from build123d import *

# Parameters (mm, degrees)
BOSS_EXTRUDE1_DEPTH              = 20
SKETCH2_R                        = 5
CUT_EXTRUDE1_DEPTH               = 10
SKETCH3_R                        = 10
CUT_EXTRUDE2_DEPTH               = 10
F_10_8_10_8_DIAMETER_HOLE1_D     = 10.8
F_10_8_10_8_DIAMETER_HOLE1_DEPTH = 5
F_10_8_10_8_DIAMETER_HOLE1_TIP   = 3.244647343
F_6_6_6_6_DIAMETER_HOLE1_D       = 6.6


with BuildPart() as part:
    # Sketch1 → Boss-Extrude1 (new body)
    with BuildSketch(Plane.XY):
        Polygon((-17, 16.25), (-17, 26.75), (17, 26.75), (17, 16.25), (30, 16.25), (30, -16.25), (-30, -16.25), (-30, 16.25), align=None)
    extrude(amount=BOSS_EXTRUDE1_DEPTH)

    # Sketch2 → Cut-Extrude1 (cut)
    with BuildSketch(Plane.XY.offset(20)):
        with Locations((0, 8.75)):
            Circle(SKETCH2_R)
    extrude(amount=-CUT_EXTRUDE1_DEPTH, mode=Mode.SUBTRACT)

    # Sketch3 → Cut-Extrude2 (cut)
    with BuildSketch(Plane(origin=(0, 0, 0), x_dir=(-1, 0, 0), z_dir=(0, 0, -1))):
        with Locations((0, 8.75)):
            Circle(SKETCH3_R)
    extrude(amount=-CUT_EXTRUDE2_DEPTH, mode=Mode.SUBTRACT)

    # Ø10.8 (10.8) Diameter Hole1
    with Locations(Plane(origin=(0, 16.25, 0), x_dir=(1, 0, 0), z_dir=(0, 1, 0))):
        with Locations((-23, -10), (23, -10)):
            Hole(F_10_8_10_8_DIAMETER_HOLE1_D / 2, depth=F_10_8_10_8_DIAMETER_HOLE1_DEPTH)
            with Locations((0, 0, -(F_10_8_10_8_DIAMETER_HOLE1_DEPTH + F_10_8_10_8_DIAMETER_HOLE1_TIP / 2))):  # 118° drill point
                Cone(0, F_10_8_10_8_DIAMETER_HOLE1_D / 2, F_10_8_10_8_DIAMETER_HOLE1_TIP, mode=Mode.SUBTRACT)

    # Ø6.6 (6.6) Diameter Hole1 (through all)
    with Locations(Plane(origin=(0, 16.25, 0), x_dir=(1, 0, 0), z_dir=(0, 1, 0))):
        with Locations((-23, -10), (23, -10)):
            Hole(F_6_6_6_6_DIAMETER_HOLE1_D / 2)


solid = part.part
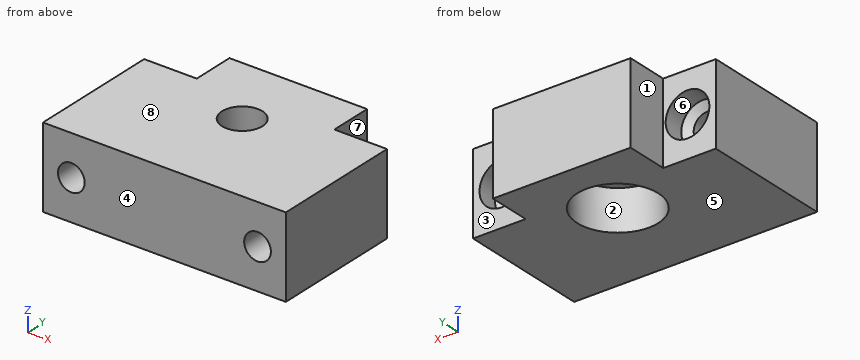
Read the model definition and answer for the solid it produces. Units are mm, in the model's axes. Face numbers are marked on the shaded views. A direction names the side the tool comes from. Give positions to 0.01 mm unless a question says otherwise; leave off trailing zeros. Write each loop counter-clockwise with the first axis right and the second up, starting at its lowest first coordinate (ties: lowest second). Pieces come first, ordered by that corner, then holes. Notation, with made-up numbers: (75.25, 9) - (107.25, 9) arc R19 ccw to (107.25, 25) - close; hole circle Ø4 at (80, -27.75). An arc over 180 degrees is marked (long way). Use CSV: the item, a comma, the result in double quotes. Start each with the question number.
Item 1: Flat-ended cylindrical pins translate along their axes: P1, Ø8.5, axis at y = 23, z = 11, coming from the +X side; P2, Ø6, axis at x = 23, z = 10, coming from the -Y side; P3, Ø9.5, axis at x = -23, z = 10, coming from the +Y side; P4, Ø6.5, axis at x = -25, z = 8, coming from the +Y side. Find the tip coordinate at first contact, or state that the pin passes through.
Item 2: The part is cut by section B-B, the plane x = 23. Give the vertices of the cut face in (y, z), and give its area (3 significant figures).
Item 3: Consider line 1 (X direction, y = -9, z = 10); line 2 (Y direction, x = 0, z = 16.75); line 3 (Z direction, x = 23, y = 12.3). Determine where each line is inside the solid, lowest interval first.
Item 4: The part is cut by section D-D, the plane y = 0. Give the vertices of the cut face in (x, z), and give its area (3 significant figures).
Item 5: The part is cut by section C-C, the plane z = 17. Give the vertices of the cut face in (x, y), and give its area (3 significant figures).
Item 6: For the marked faces 1, 2, 3 and 4, determine the directions among +Z, -Z, +X, -X, +Y, -Y from which every point of the face is accessible in a straight line to the end or side of a thin tool.
Item 7: The part is cut by section A-A, the plane y = 8.75. Give the vertices of the cut face in (x, z), and give its area (3 significant figures).
Item 8: The mould has two halves that part along Z. Classify the marked faces 5, 6, 7 and 8: pulls with the +Z half, pulls with the -Z half, needs draft (parallel to the pull), parting line crosses it, or undercut.
Taken from the geometry:
1,P1,"x = 17"
1,P2,"through"
1,P3,"y = 10.86"
1,P4,"y = 16.25"
2,outline,"(-16.25, 0) - (16.25, 0) - (16.25, 4.6) - (11.25, 4.6) - (9.99, 6.7) - (-16.25, 6.7) - close; (-16.25, 13.3) - (9.99, 13.3) - (11.25, 15.4) - (16.25, 15.4) - (16.25, 20) - (-16.25, 20) - close"
2,area,"412 mm2"
3,line 1,"-30 to -26.3, -19.7 to 19.7, 26.3 to 30"
3,line 2,"-16.25 to 3.75, 13.75 to 26.75"
3,line 3,"0 to 4.6, 15.4 to 20"
4,outline,"(-30, 0) - (-4.84, 0) - (-4.84, 10) - (4.84, 10) - (4.84, 0) - (30, 0) - (30, 20) - (-30, 20) - close; hole circle Ø6.6 at (-23, 10); hole circle Ø6.6 at (23, 10)"
4,area,"1,030 mm2"
5,outline,"(-30, -16.25) - (30, -16.25) - (30, 16.25) - (17, 16.25) - (17, 26.75) - (-17, 26.75) - (-17, 16.25) - (-30, 16.25) - close; hole circle Ø10 at (0, 8.75)"
5,area,"2,230 mm2"
6,face 1,"+Z, -Z, -X, +Y"
6,face 2,"-Z"
6,face 3,"+Z, -Z, +X, +Y"
6,face 4,"+Z, -Z, +X, -X, -Y"
7,outline,"(-30, 0) - (-10, 0) - (-10, 10) - (-5, 10) - (-5, 20) - (-30, 20) - close; (5, 10) - (10, 10) - (10, 0) - (30, 0) - (30, 20) - (5, 20) - close; hole circle Ø6.6 at (-23, 10); hole circle Ø6.6 at (23, 10)"
7,area,"832 mm2"
8,face 5,"pulls with the -Z half"
8,face 6,"undercut"
8,face 7,"needs draft"
8,face 8,"pulls with the +Z half"
